Build history of the part. All positions in model axes, mm. A direction names the side the tool comes from. Round coordinates to 2 decimals unless told otherwise and drop trailing zeros. Write each loop counter-clockwise with the first axis right and the second up, starting at its lowest first coordinate (ties: lowest second). Pieces come first, ordered by that corner, then holes. Notation, with made-up numbers: M -39.5,-2.5 L -21.5,-2.5 A32 cw -21.5,34.5 Z; hole C 66,40.25 d5. An arc over 180 degrees is marked long. Write item = value, one per line.
from build123d import *

# Parameters (mm, degrees)
F0_R     = 22
F1_DEPTH = 25
F2_R     = 5.5
F3_R     = 18.5
F4_DEPTH = 21
F5_R     = 1.5


with BuildPart() as f1:
    # F0 (on Top) → F1 (new body)
    with BuildSketch(Plane.XY):
        Circle(F0_R)
    extrude(amount=F1_DEPTH)

    # F2
    f2_edges = [f1.edges().sort_by_distance(p)[0] for p in [
        (-22, 0, 25),
    ]]
    fillet(f2_edges, radius=F2_R)

    # F3 (on Top) → F4 (cut)
    with BuildSketch(Plane.XY):
        Circle(F3_R)
    extrude(amount=F4_DEPTH, mode=Mode.SUBTRACT)

    # F5
    f5_edges = [f1.edges().sort_by_distance(p)[0] for p in [
        (-18.5, 0, 21),
    ]]
    fillet(f5_edges, radius=F5_R)


solid = f1.part
1. Band-saw the part on A-A (y = 0). List the corners of the cut face in (x, z).
Responses:
outline = M -22,0 L -18.5,0 L -18.5,19.5 A1.5 cw -17,21 L 17,21 A1.5 cw 18.5,19.5 L 18.5,0 L 22,0 L 22,19.5 A5.5 ccw 16.5,25 L -16.5,25 A5.5 ccw -22,19.5 Z
2. Probe probe 1 along Y at (x, z) = (0.5, 7.75); probe 2 along Z at (x, y) = (-5, -5); probe 3 along X at (y, z) = (-1.5, 16). List the from-to ranges inside material, lowest first.
Responses:
probe_1 = -21.99 to -18.49, 18.49 to 21.99
probe_2 = 21 to 25
probe_3 = -21.95 to -18.44, 18.44 to 21.95
3. Mould opens along Y. For faces 1 (the face through (0, 0, 21)), 2 (the face through (-4.769, -21.477, 9.614)), 3 (the face through (-5, 18, 0)) say: pulls with the +Y half, pulls with the -Y half, needs draft (parallel to the pull), parting line crosses it, or undercut.
Responses:
face_1 = undercut
face_2 = parting line crosses it
face_3 = needs draft
4. Tool access for faces 4 (the face through (0, 0, 25)), 5 (the face through (-4.01, -18.06, 9.61)): list every direction of +Z, -Z, +X, -X, +Y, -Y with a clear straight run to the whole face (end or side of a thin tool).
Responses:
face_4 = +Z, +X, -X, +Y, -Y
face_5 = -Z
5. Flat gauge pins, fed straight in: pin 1 (5 mm diameter, centred on x = 0.5, y = 12, fed in from -Z); pin 2 (8 mm diameter, centred on y = -15.5, z = 17, fed in from +X) (3 decimals); pin 3 (12 mm diameter, centred on x = -3.5, z = 5.5, fed in from -Y). Where does each tip first touch, or does it go through?
Responses:
pin_1 = 21
pin_2 = 18.755
pin_3 = -22
6. Band-saw the part on B-B (z = 5.5). List the corners of the cut face in (x, y), plus the area to 3 significant figures.
Responses:
outline = C 0,0 d44; hole C 0,0 d37
area = 445 mm²
